Input: part model. Units: mm. Frame: model coordinates. Face numbers are marked on the shaded views. Coordinates: 2 decimals unless noted, no trailing zeros. Write each loop counter-clockwise with the first axis right and the second up, starting at its lowest first coordinate (ties: lowest second). Pieces come first, ordered by that corner, then holes. Notation, with made-up numbers: (10.5, 28) - (27.5, 28) arc R15 cw to (27.5, 47) - close; hole circle Ø4 at (-23, 43). An arc over 180 degrees is marked (long way). Use a Markdown table: item, result. Add a question column.
Q1. Material intervals for probe 1 along Z at (x, y) = (11, 0.4); probe 2 along Z at (x, y) = (11, 0.2); probe 3 along Y at (x, z) = (9, 4.25), sorted ascending. Write a range as from..to.
Q2. Mould query, pull axis X, two halves, no side actions, for the marked faces 1, 2 and 3. Classes: released by +X, released by -X, zero draft, split by the parting line, or undercut.
Q3. Section query A-A (x = 11). Return the cut outline in (y, z).
Q4. Pin query (flat end, axial travel): P1, Ø3, axis at x = 11, z = -5, coming from the -Y side; P2, Ø1.8, axis at x = 11, z = 5, coming from the -Y side. Return the tip coordinate at first contact, or that it passes through.
from build123d import *

# Parameters (mm, degrees)
SKETCH_1_W               = 4
SKETCH_1_H               = 16
EXTRUDE_1_DEPTH          = 3
EXTRUDE_1_TAPER          = 10
EXTRUDE_3_DEPTH          = 1.5
EXTRUDE_4_DEPTH          = 16
CUT_EXTRUDE_1_REACH      = 19.263
CUT_EXTRUDE_1_END_RADIUS = 15
SKETCH_6_R               = 1.1
CUT_EXTRUDE_2_DEPTH      = 18.066048222
CHAMFER_1_SIZE           = 1
FILLET_2_R               = 1
FILLET_3_R               = 0.5


with BuildPart() as part:
    # Sketch 1 → Extrude 1 (new body)
    with BuildSketch(Plane(origin=(0, 0, 0), x_dir=(1, 0, 0), z_dir=(0, 1, 0))):
        with Locations((5.671019058, 0)):
            Rectangle(SKETCH_1_W, SKETCH_1_H)
    extrude(amount=EXTRUDE_1_DEPTH, taper=EXTRUDE_1_TAPER)



with BuildPart() as body_2:
    # Sketch 2 → Extrude 3 (new body)
    with BuildSketch(Plane(origin=(0, 0, 0), x_dir=(1, 0, 0), z_dir=(0, 1, 0))):
        with BuildLine():
            Line((7.671019058, 8), (12.68857754, 8))
            ThreePointArc((12.68857754, 8), (15, 0), (12.68857754, -8))
            Line((12.68857754, -8), (7.671019058, -8))
            Line((7.671019058, -8), (7.671019058, 8))
        make_face()
    extrude(amount=EXTRUDE_3_DEPTH)


with BuildPart() as part_1:
    add(part.part)

    add(body_2.part)  # Extrude 4 merges body 2
    # Sketch 3 → Extrude 4 (add)
    with BuildSketch(Plane.XY.offset(8)):
        Polygon((7.671019058, 1.5), (7.406528587, 1.5), (7.671019058, 0), align=None)
    extrude(amount=-EXTRUDE_4_DEPTH)

    # Cut-Extrude 1: up to this cylinder (the profile starts inside it)
    cut_extrude_1_end = Plane(origin=(0, 1, 0), z_dir=(0, -1, 0)) * Cylinder(CUT_EXTRUDE_1_END_RADIUS, 69.526, mode=Mode.PRIVATE)
    # Sketch 5 → Cut-Extrude 1 (cut, up to the surface)
    with BuildSketch(Plane(origin=(0, 0, 0), x_dir=(0, 0, -1), z_dir=(1, 0, 0)), mode=Mode.PRIVATE) as cut_extrude_1_sk1:
        Polygon((-8, 0), (-8, 1.5), (-7.735509529, 1.5), align=None)
    cut_extrude_1_tool1 = extrude(cut_extrude_1_sk1.sketch, amount=CUT_EXTRUDE_1_REACH, mode=Mode.PRIVATE) & cut_extrude_1_end
    add(cut_extrude_1_tool1.solids().sort_by_distance((0, 1, 7.911837))[0], mode=Mode.SUBTRACT)
    # Sketch 5 → Cut-Extrude 1 (cut, up to the surface)
    with BuildSketch(Plane(origin=(0, 0, 0), x_dir=(0, 0, -1), z_dir=(1, 0, 0)), mode=Mode.PRIVATE) as cut_extrude_1_sk2:
        Polygon((7.735509529, 1.5), (8, 0), (8, 1.5), align=None)
    cut_extrude_1_tool2 = extrude(cut_extrude_1_sk2.sketch, amount=CUT_EXTRUDE_1_REACH, mode=Mode.PRIVATE) & cut_extrude_1_end
    add(cut_extrude_1_tool2.solids().sort_by_distance((0, 1, -7.911837))[0], mode=Mode.SUBTRACT)

    # Sketch 6 → Cut-Extrude 2 (cut, through all)
    with BuildSketch(Plane(origin=(0, 1.5, 0), x_dir=(1, 0, 0), z_dir=(0, 1, 0))):
        with Locations(Location((11, 5, 0), (0, 0, 180))):
            Circle(SKETCH_6_R)
        with Locations(Location((11, -5, 0), (0, 0, 180))):
            Circle(SKETCH_6_R)
    extrude(amount=-CUT_EXTRUDE_2_DEPTH, mode=Mode.SUBTRACT)

    # Chamfer 1
    chamfer_1_edges = [part_1.edges().sort_by_distance(p)[0] for p in [
        (12.1, 1.5, -5),
        (12.1, 1.5, 5),
    ]]
    chamfer(chamfer_1_edges, length=CHAMFER_1_SIZE)

    # Fillet 2
    fillet_2_edges = [part_1.edges().sort_by_distance(p)[0] for p in [
        (7.406528587, 1.5, 0),
    ]]
    fillet(fillet_2_edges, radius=FILLET_2_R)

    # Fillet 3
    fillet_3_edges = [part_1.edges().sort_by_distance(p)[0] for p in [
        (4.2, 3, 0),
        (5.671019058, 3, 7.471019058),
        (7.142038116, 3, 0),
        (3.935509529, 1.5, 7.735509529),
        (3.935509529, 1.5, -7.735509529),
        (5.671019058, 3, -7.471019058),
    ]]
    fillet(fillet_3_edges, radius=FILLET_3_R)


solid = part_1.part
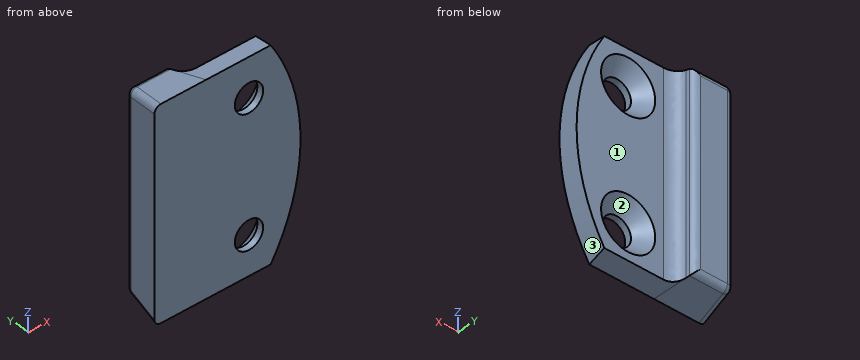
Values follow:
| question | item | result |
|---|---|---|
| 1 | probe 1 | -7.93..-6.1, -3.9..3.9, 6.1..7.93 |
| 1 | probe 2 | -7.96..-6.1, -3.9..3.9, 6.1..7.96 |
| 1 | probe 3 | 0..1.5 |
| 2 | face 1 | zero draft |
| 2 | face 2 | undercut |
| 2 | face 3 | released by +X |
| 3 | outline | (0, -8) - (1.5, -7.74) - (1.5, -7.1) - (0.5, -6.1) - (0, -6.1) - close; (0, -3.9) - (0.5, -3.9) - (1.5, -2.9) - (1.5, 2.9) - (0.5, 3.9) - (0, 3.9) - close; (0, 6.1) - (0.5, 6.1) - (1.5, 7.1) - (1.5, 7.74) - (0, 8) - close |
| 4 | P1 | y = 0 |
| 4 | P2 | through |
